Build history of the part. All positions in model axes, mm. Face numbers are marked on the shaded views. Give positions to 0.01 mm unless a question says otherwise; leave off trailing zeros. Write each loop counter-clockwise with the first axis right and the second up, starting at its lowest first coordinate (ties: lowest second). Pieces come first, ordered by that corner, then holes. Notation, with made-up numbers: (-13.75, -34) - (37.25, -34) arc R28 ccw to (37.25, -2) - close; hole circle Ø6 at (24, 32.5). An arc over 180 degrees is marked (long way). Use one line per item in the form item = value. Start each with the question number.
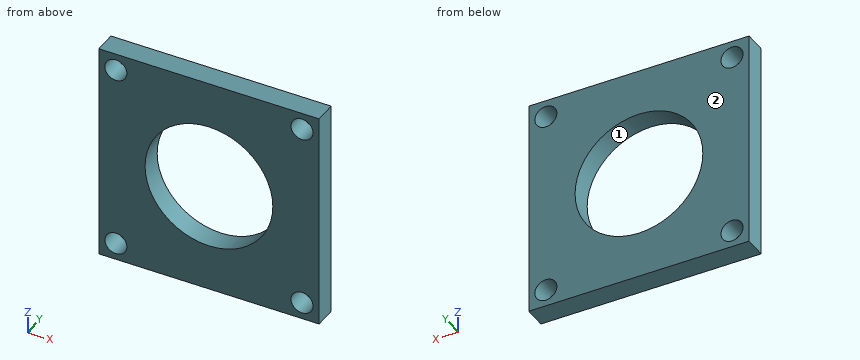
Autodesk Inventor part; units mm, degrees
ref_plane "YZ Plane" through (0, 0, 0) normal (1, 0, 0) x (0, 1, 0)
ref_plane "XZ Plane" through (0, 0, 0) normal (0, 1, 0) x (-1, 0, 0)
ref_plane "XY Plane" through (0, 0, 0) normal (0, 0, 1) x (1, 0, 0)
sketch "Skizze1" plane through (0, 0, 0) normal (0, 1, 0) x (-1, 0, 0)
  line L0 (-25, 25) -> (25, 25)
  line L1 (25, 25) -> (25, -25)
  line L2 (25, -25) -> (-25, -25)
  line L3 (-25, -25) -> (-25, 25)
  line L4 (-25, 25) -> (25, -25) construction
  line L5 (25, 25) -> (-25, -25) construction
  point P0 (0, 0)
  dimension "d0" = 50
  dimension "d1" = 50
extrude "Extrusion1" add sketch "Skizze1" along normal blind 5
sketch "Skizze2" plane through (0, 5, 0) normal (0, 1, 0) x (1, 0, 0)
  point P0 (0, 0)
  point P1 (0, 0)
hole "Bohrung1" at (0, 5, 0) direction (0, -1, 0) diameter 29 depth 5
sketch "Skizze3" plane through (0, 5, 0) normal (0, 1, 0) x (1, 0, 0)
  line L0 (25, 25) -> (-25, 25)
  line L1 (0, 25) -> (0, -25) construction
  line L2 (-25, -25) -> (25, -25)
  line L3 (25, -25) -> (25, 25)
  line L4 (25, 0) -> (-25, 0) construction
  line L5 (-25, 25) -> (-25, -25)
  point P0 (0, 0)
  point P1 (-21.124, -21.124)
  point P2 (-21.124, 21.124)
  point P3 (21.124, -21.124)
  point P4 (21.124, 21.124)
  dimension "d18" = 42.248
  dimension "d19" = 42.248
hole "Bohrung2" at (-21.124, 5, 21.124) at (-21.124, 5, -21.124) at (21.124, 5, 21.124) at (21.124, 5, -21.124) direction (0, -1, 0) diameter 5 depth 5
properties part number "thickshield_cylinder"
(1) Wall check: line 1 (Z direction, x = 21, y = 3.4); line 2 (X direction, y = 3.1, z = 21.5); line 3 (X direction, y = 3.5, z = 19.5). Give the ranges that are in metal, low to high. Write a range as from..to.
(2) Cut at A-A, the plane z = 0. Give the cut face in (x, y), then the cut area to 3 significant figures.
(3) Cut at B-B, the plane x = 0. Give the cut face in (y, z), then the cut area to 3 significant figures.
(4) Two-plate mould, pull along X, no slides. Class the marked faces 1 and 2: +X half, -X half, draft (parallel to the pull), parting line (faces both ways), or undercut.
(5) Cut at C-C, the plane z = -20. Give the cut face in (x, y).
(6) Cut at D-D, the plane y = 4.15. Give the cut face in (x, z), then the cut area to 3 significant figures.
Solution:
q1.line_1 = -25..-23.62, -18.63..18.63, 23.62..25
q1.line_2 = -25..-23.6, -18.65..18.65, 23.6..25
q1.line_3 = -25..-23.02, -19.22..19.22, 23.02..25
q2.outline = (-25, 0) - (-14.5, 0) - (-14.5, 5) - (-25, 5) - close; (14.5, 0) - (25, 0) - (25, 5) - (14.5, 5) - close
q2.area = 105 mm2
q3.outline = (0, -25) - (5, -25) - (5, -14.5) - (0, -14.5) - close; (0, 14.5) - (5, 14.5) - (5, 25) - (0, 25) - close
q3.area = 105 mm2
q4.face_1 = undercut
q4.face_2 = draft
q5.outline = (-25, 0) - (-23.36, 0) - (-23.36, 5) - (-25, 5) - close; (-18.89, 0) - (18.89, 0) - (18.89, 5) - (-18.89, 5) - close; (23.36, 0) - (25, 0) - (25, 5) - (23.36, 5) - close
q6.outline = (-25, -25) - (25, -25) - (25, 25) - (-25, 25) - close; hole circle Ø5 at (-21.12, -21.12); hole circle Ø5 at (-21.12, 21.12); hole circle Ø29 at (0, 0); hole circle Ø5 at (21.12, -21.12); hole circle Ø5 at (21.12, 21.12)
q6.area = 1,760 mm2
